```python
from build123d import *

# Parameters (mm, degrees)
SKETCH1_W                    = 100
SKETCH1_H                    = 60
BOSS_EXTRUDE1_DEPTH          = 3.175
CUT_EXTRUDE1_DEPTH           = 3.175
TAP_DRILL_FOR_M12X1_5_TAP1_D = 10.5


with BuildPart() as part:
    # Sketch1 → Boss-Extrude1 (new body)
    with BuildSketch(Plane(origin=(0, 0, 0), x_dir=(1, 0, 0), z_dir=(0, 1, 0))):
        with Locations((50, -30)):
            Rectangle(SKETCH1_W, SKETCH1_H)
    extrude(amount=BOSS_EXTRUDE1_DEPTH)

    # Sketch2 → Cut-Extrude1 (cut)
    with BuildSketch(Plane(origin=(0, 3.175, 0), x_dir=(1, 0, 0), z_dir=(0, 1, 0))):
        Polygon((3.175, -25), (3.175, -35), (3.175, -60), (0, -60), (0, -45), (0, -25), align=None)
        Polygon((100, -25), (96.825, -25), (96.825, -35), (96.825, -60), (100, -60), (100, -45), align=None)
    extrude(amount=-CUT_EXTRUDE1_DEPTH, mode=Mode.SUBTRACT)

    # Tap Drill for M12x1.5 Tap1 (through all)
    with Locations(Plane(origin=(0, 3.175, 0), x_dir=(1, 0, 0), z_dir=(0, 1, 0))):
        with Locations((50, -30)):
            Hole(TAP_DRILL_FOR_M12X1_5_TAP1_D / 2)


solid = part.part
```
The model under review builds one solid part; all positions refer to its coordinate system, in mm. A direction names the side the tool comes from. Coordinates: 2 decimals unless noted, no trailing zeros. Order: outer loops, then holes, each group sorted by start corner. A loop starts at its lowest first (then second) coordinate and runs counter-clockwise, first axis right, second up. Notation, with made-up numbers: (-27.75, -18) -> (8.25, -18) arc R21 ccw to (8.25, 1) -> close; hole circle Ø7 at (38.25, 21.25). An arc over 180 degrees is marked (long way). Answer in a Markdown table with one row per item. Add a question column.
Item 1: To check wall thickness, follow probe 1 along Z at (x, y) = (50, 1.35); probe 2 along X at (y, z) = (0.65, 30) (3 decimals); probe 3 along X at (y, z) = (2.2, 37.5) (3 decimals). State the ranges of each line that lie inside material, in increasing order.
Item 2: Mouldability with a two-part tool opening along X and no side actions: class faces 1 (the flat face through (96.825, 2, 42)), 2 (the flat face through (49, 2, 60)), 3 (the cylindrical face through (54.17, 1.57, 33.19)) as +X half, -X half, draft (parallel to the pull), parting line (faces both ways), or undercut.
Item 3: We need section D-D on z = 51.5. Write out the cut boundary in (x, y) (3 decimals).
Item 4: Clearance check with flat-ended pins moving along their axes: pin 1 (1 mm diameter, centred on y = 2, z = 42.5, fed in from -X) (3 decimals); pin 2 (1 mm diameter, centred on x = 99, y = 2, fed in from +Z). State where each tip first meets the part, or that it passes through.
Item 5: Machinability: for faces 4 (the flat face through (98, 2, 25)), 5 (the flat face through (3.175, 2, 43)), 6 (the flat face through (49, 3.175, 23)), which of the approach directions +Z, -Z, +X, -X, +Y, -Y give a long, thin tool a straight path to every point of the face, cutting with its end or side? Answer none if there is none.
Item 6: We need section A-A on z = 30. Write out the cut boundary in (x, y) (3 decimals), plus the area to 3 significant figures.
Item 7: We need section C-C on y = 2. Write out the cut boundary in (x, z) (3 decimals).
Item 8: We need section B-B on x = 50. Write out the cut boundary in (y, z) (3 decimals), plus the area to 3 significant figures.
Final values:
| question | item | result |
|---|---|---|
| 1 | probe 1 | z = 0 to 24.75, 35.25 to 60 |
| 1 | probe 2 | x = 3.175 to 44.75, 55.25 to 96.825 |
| 1 | probe 3 | x = 3.175 to 96.825 |
| 2 | face 1 | +X half |
| 2 | face 2 | draft |
| 2 | face 3 | undercut |
| 3 | outline | (3.175, 0) -> (96.825, 0) -> (96.825, 3.175) -> (3.175, 3.175) -> close |
| 4 | pin 1 | stops at x = 3.175 |
| 4 | pin 2 | stops at z = 25 |
| 5 | face 4 | +Z, +X, +Y, -Y |
| 5 | face 5 | +Z, -X, +Y, -Y |
| 5 | face 6 | +Z, -Z, +X, -X, +Y |
| 6 | outline | (3.175, 0) -> (44.75, 0) -> (44.75, 3.175) -> (3.175, 3.175) -> close; (55.25, 0) -> (96.825, 0) -> (96.825, 3.175) -> (55.25, 3.175) -> close |
| 6 | area | 264 mm2 |
| 7 | outline | (0, 0) -> (100, 0) -> (100, 25) -> (96.825, 25) -> (96.825, 60) -> (3.175, 60) -> (3.175, 25) -> (0, 25) -> close; hole circle Ø10.5 at (50, 30) |
| 8 | outline | (0, 0) -> (3.175, 0) -> (3.175, 24.75) -> (0, 24.75) -> close; (0, 35.25) -> (3.175, 35.25) -> (3.175, 60) -> (0, 60) -> close |
| 8 | area | 157 mm2 |
